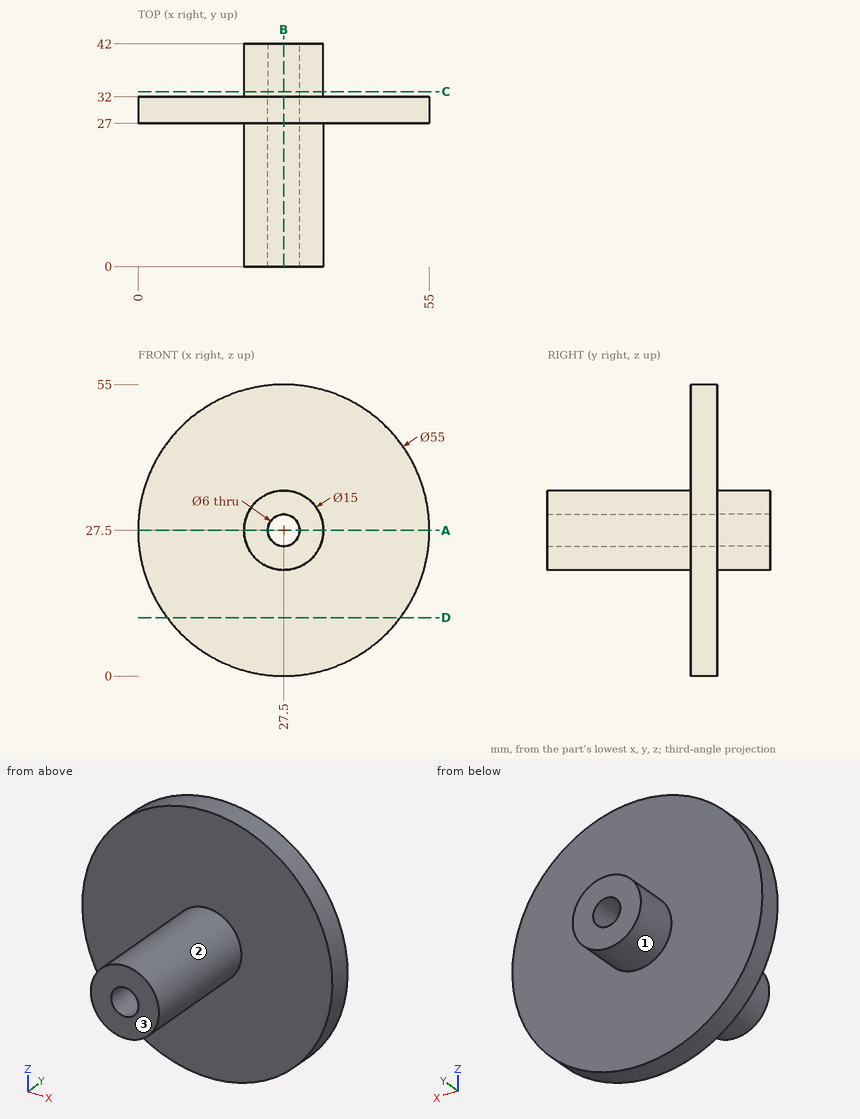
Study the drawing (mm; zero at the part's minimum x, y, z) and answer. A direction names the side the tool comes from. Round coordinates to 2 decimals unless told otherwise and drop trailing zeros. Order: outer loops, then holes, each group sorted by start corner. A loop starts at its lowest first (then second) coordinate and runs counter-clockwise, first axis right, second up. Notation, with made-up numbers: (-8.5, 83) -> (8.5, 83) arc R16 ccw to (8.5, 106) -> close; hole circle Ø8 at (42.25, 79). An arc over 180 degrees is marked (long way). Write each question's results on one line, items separated by ' | '. Start each with the question number.
Q1. Find section C-C (y = 33). Determine the outline of the cut face in (x, z), then the cut area to 3 significant figures.
Q2. Which of the six approach directions +Z, -Z, +X, -X, +Y, -Y give full straight-line access (tool end or side, diameter ignored) to the marked faces 1, 2 and 3?
Q3. Find section B-B (x = 27.5). Determine the outline of the cut face in (y, z), then the cut area to 3 significant figures.
Q4. Find section D-D (z = 11). Determine the outline of the cut face in (x, y).
Q5. Find section A-A (z = 27.5). Determine the outline of the cut face in (x, y), then the cut area to 3 significant figures.
Q6. Straight lines are drawn through the part: probe 1 along Z at (x, y) = (27.5, 10); probe 2 along Y at (x, z) = (43, 40). For each, find the intervals that lie inside material, in ascending order. Write a range as from..to.
Q7. Each of these flat-tipped pins is pushed along its axis until it touches: pin 1 (4 mm diameter, centred on x = 25, y = 16.5, fed in from +Z); pin 2 (2 mm diameter, centred on y = 23, z = 34, fed in from +X); pin 3 (1.5 mm diameter, centred on x = 25.5, y = 4.5, fed in from +Z). Where does it stop, or does it pass through?
Worked answers:
1) outline: circle Ø15 at (27.5, 27.5); hole circle Ø6 at (27.5, 27.5) | area: 148 mm2
2) face 1: +Y | face 2: -Y | face 3: +Z, -Z, +X, -X, -Y
3) outline: (0, 20) -> (27, 20) -> (27, 0) -> (32, 0) -> (32, 20) -> (42, 20) -> (42, 24.5) -> (0, 24.5) -> close; (0, 30.5) -> (42, 30.5) -> (42, 35) -> (32, 35) -> (32, 55) -> (27, 55) -> (27, 35) -> (0, 35) -> close | area: 578 mm2
4) outline: (5.5, 27) -> (49.5, 27) -> (49.5, 32) -> (5.5, 32) -> close
5) outline: (0, 27) -> (20, 27) -> (20, 0) -> (24.5, 0) -> (24.5, 42) -> (20, 42) -> (20, 32) -> (0, 32) -> close; (30.5, 0) -> (35, 0) -> (35, 27) -> (55, 27) -> (55, 32) -> (35, 32) -> (35, 42) -> (30.5, 42) -> close | area: 578 mm2
6) probe 1: z = 20..24.5, 30.5..35 | probe 2: y = 27..32
7) pin 1: stops at z = 34.98 | pin 2: stops at x = 32.6 | pin 3: stops at z = 34.9
